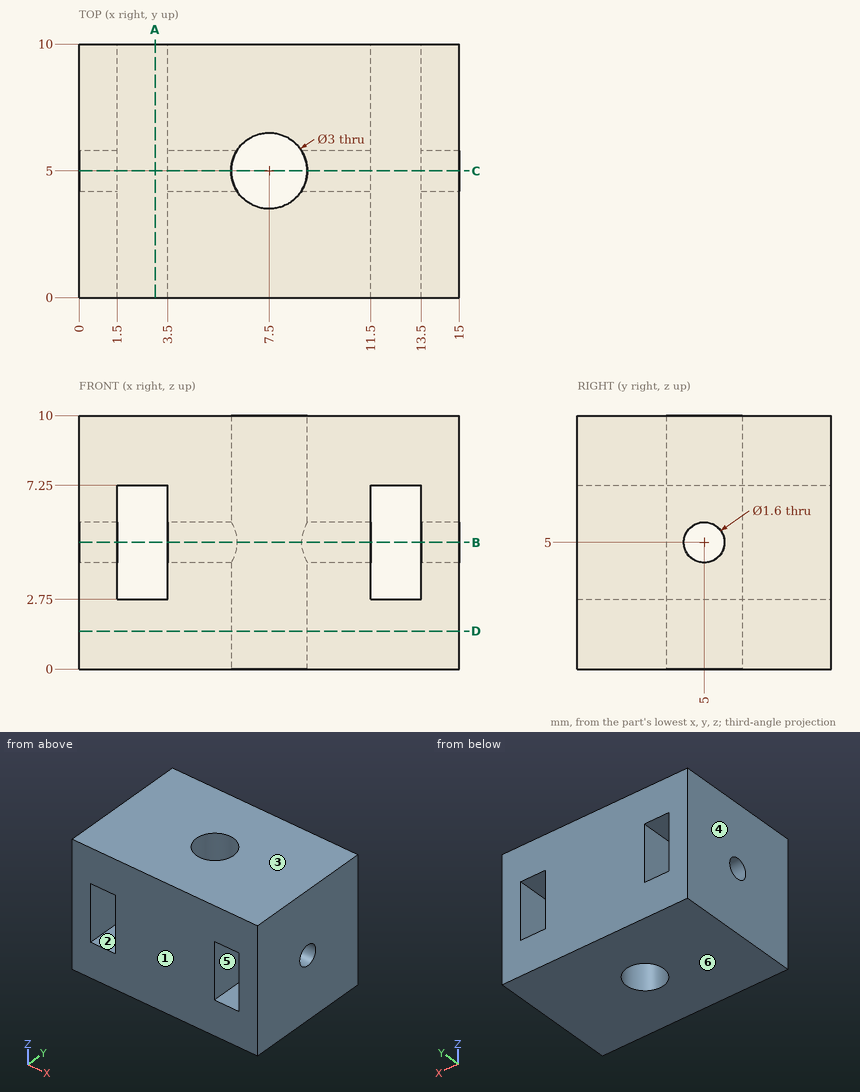
Study the drawing (mm; zero at the part's minimum x, y, z) and answer. A direction names the side the tool comes from. Round coordinates to 2 decimals unless told otherwise and drop trailing zeros. Loops run counter-clockwise (first coordinate to the right, second up) from the corner with the lowest first, then second, coordinate; pieces in that order, holes last. Notation, with made-up numbers: M 61.25,-8 L 97.25,-8 A14 ccw 97.25,1 Z; hole C 79.25,-12 d1. An arc over 180 degrees is marked long. One line per question, with ' | ' between items.
Q1. The mould has two halves that part along Z. Classify the marked faces 3, 4, 5 and 6: +Z half, -Z half, draft (parallel to the pull), parting line (faces both ways), or undercut.
Conclusion:
face 3: +Z half | face 4: draft | face 5: undercut | face 6: -Z half
Q2. Consider line 1 along X through (y, z) = (2, 3.5); line 2 along Z through (x, y) = (2.75, 0.5); line 3 along Z through (x, y) = (0.6, 5). Determine where each line is inside the solid, lowest interval first. Write a range as from..to.
Conclusion:
line 1: x = 0..1.5, 3.5..11.5, 13.5..15 | line 2: z = 0..2.75, 7.25..10 | line 3: z = 0..4.2, 5.8..10
Q3. This flat-tipped pin is pushed along its axis until it touches: pin 1 Ø1 at (y, z) = (5, 5) entering from -X. Where does it stop, or does it pass through?
Conclusion:
pin 1: passes through
Q4. A tool of negligible diameter and unlimited length cuts with its end or side. For the marked faces 1 and 2, from which of +Z, -Z, +X, -X, +Y, -Y can it reach the whole face along a straight path? Write none if from no direction.
Conclusion:
face 1: +Z, -Z, +X, -X, -Y | face 2: +Y, -Y
Q5. Find section D-D, the plane z = 1.5. Give the vertices of the cut face in (x, y).
Conclusion:
outline: M 0,0 L 15,0 L 15,10 L 0,10 Z; hole C 7.5,5 d3
Q6. Find section B-B, the plane z = 5. Give the vertices of the cut face in (x, y), then the cut area to 3 significant figures.
Conclusion:
outline: M 0,0 L 1.5,0 L 1.5,4.2 L 0,4.2 Z; M 0,5.8 L 1.5,5.8 L 1.5,10 L 0,10 Z; M 3.5,0 L 11.5,0 L 11.5,4.2 L 8.77,4.2 A1.5 cw 6.23,4.2 L 3.5,4.2 Z; M 3.5,5.8 L 6.23,5.8 A1.5 cw 8.77,5.8 L 11.5,5.8 L 11.5,10 L 3.5,10 Z; M 13.5,0 L 15,0 L 15,4.2 L 13.5,4.2 Z; M 13.5,5.8 L 15,5.8 L 15,10 L 13.5,10 Z | area: 89.9 mm2
Q7. Find section C-C, the plane y = 5. State how many separate pieces and enclosed holes the cut face has, then the cut area to 3 significant figures.
Conclusion:
separate pieces: 4 | enclosed holes: 0 | area: 89.2 mm2
Q8. Find section A-A, the plane x = 3. Give the vertices of the cut face in (y, z).
Conclusion:
outline: M 0,0 L 10,0 L 10,2.75 L 0,2.75 Z; M 0,7.25 L 10,7.25 L 10,10 L 0,10 Z
